from build123d import *

# Parameters (mm, degrees)
SKETCH1_W                     = 10.4775
SKETCH1_H                     = 12.7
SKETCH1_R                     = 2
SKETCH1_W_2                   = 13.97
BOSS_EXTRUDE1_DEPTH           = 7.9375
SKETCH2_W                     = 13.97
SKETCH2_H                     = 12.7
BOSS_EXTRUDE2_DEPTH           = 11.1125
CUT_EXTRUDE1_DEPTH            = 11.43
SKETCH4_R                     = 1.143
CUT_EXTRUDE2_DEPTH            = 32.637086722
CBORE_FOR_M4_SHCS1_AT_2_COUNT = 2
CBORE_FOR_M4_SHCS1_AT_2_PITCH = 24.4475
SKETCH8_R                     = 3
SKETCH8_R_2                   = 1.143
CUT_EXTRUDE3_DEPTH            = 32.637086722


with BuildPart() as part:
    # Sketch1 → Boss-Extrude1 (new body)
    # profile 1 of 5: a face of its own
    with BuildSketch(Plane.XY):
        with Locations((12.22375, 0)):
            Rectangle(SKETCH1_W, SKETCH1_H)
        with Locations((12.22375, 0)):
            Circle(SKETCH1_R, mode=Mode.SUBTRACT)
    # profile 2 of 5: a face of its own
    with BuildSketch(Plane.XY):
        Rectangle(SKETCH1_W_2, SKETCH1_H)
    # profile 3 of 5: a face of its own
    with BuildSketch(Plane.XY):
        with Locations((-12.22375, 0)):
            Rectangle(SKETCH1_W, SKETCH1_H)
        with Locations((-12.22375, 0)):
            Circle(SKETCH1_R, mode=Mode.SUBTRACT)
    # profile 4 of 5: a face of its own
    with BuildSketch(Plane.XY):
        with Locations((12.22375, 0)):
            Circle(SKETCH1_R)
    # profile 5 of 5: a face of its own
    with BuildSketch(Plane.XY):
        with Locations((-12.22375, 0)):
            Circle(SKETCH1_R)
    extrude(amount=BOSS_EXTRUDE1_DEPTH)

    # Sketch2 → Boss-Extrude2 (add)
    with BuildSketch(Plane.XY.offset(7.9375)):
        Rectangle(SKETCH2_W, SKETCH2_H)
    extrude(amount=BOSS_EXTRUDE2_DEPTH)

    # Sketch3 → Cut-Extrude1 (cut)
    with BuildSketch(Plane(origin=(6.985, 0, 0), x_dir=(0, 0, -1), z_dir=(1, 0, 0))):
        with BuildLine():
            ThreePointArc((-13.49375, 3), (-16.49375, 0), (-13.49375, -3))
            Line((-13.49375, -3), (-13.49375, -1.143))
            ThreePointArc((-13.49375, -1.143), (-14.63675, 0), (-13.49375, 1.143))
            Line((-13.49375, 1.143), (-13.49375, 3))
        make_face()
        with BuildLine():
            Line((-13.49375, -1.143), (-13.49375, -3))
            ThreePointArc((-13.49375, -3), (-11.372429656, -2.121320344), (-10.49375, 0))
            ThreePointArc((-10.49375, 0), (-11.372429656, 2.121320344), (-13.49375, 3))
            Line((-13.49375, 3), (-13.49375, 1.143))
            ThreePointArc((-13.49375, 1.143), (-12.685526949, 0.808223051), (-12.35075, 0))
            ThreePointArc((-12.35075, 0), (-12.685526949, -0.808223051), (-13.49375, -1.143))
        make_face()
        with BuildLine():
            ThreePointArc((-13.49375, 1.143), (-14.63675, 0), (-13.49375, -1.143))
            Line((-13.49375, -1.143), (-13.49375, 1.143))
        make_face()
        with BuildLine():
            Line((-13.49375, 1.143), (-13.49375, -1.143))
            ThreePointArc((-13.49375, -1.143), (-12.685526949, -0.808223051), (-12.35075, 0))
            ThreePointArc((-12.35075, 0), (-12.685526949, 0.808223051), (-13.49375, 1.143))
        make_face()
    extrude(amount=-CUT_EXTRUDE1_DEPTH, mode=Mode.SUBTRACT)

    # Sketch4 → Cut-Extrude2 (cut, through all)
    with BuildSketch(Plane(origin=(6.985, 0, 0), x_dir=(0, 0, -1), z_dir=(1, 0, 0))):
        with Locations((-13.49375, 0)):
            Circle(SKETCH4_R)
    extrude(amount=-CUT_EXTRUDE2_DEPTH, mode=Mode.SUBTRACT)

    # Sketch6 → CBORE for M4 SHCS1 (revolve, cut)
    with BuildSketch(Plane(origin=(12.22375, 0, 7.9375), x_dir=(0, -1, 0), z_dir=(1, 0, 0))):
        Polygon((0, 0), (0, 7.9375), (2.25, 7.9375), (2.25, 4), (4, 4), (4, 0.025), (4.025, 0), align=None)
    cbore_for_m4_shcs1 = revolve(axis=Axis((12.22375, 0, 14.2875), (0, 0, -1)), mode=Mode.SUBTRACT)

    # CBORE for M4 SHCS1 at 2: CBORE for M4 SHCS1 ×2
    with Locations(*[(-i * CBORE_FOR_M4_SHCS1_AT_2_PITCH, 0, 0) for i in range(1, CBORE_FOR_M4_SHCS1_AT_2_COUNT)]):
        add(cbore_for_m4_shcs1, mode=Mode.SUBTRACT)

    # Sketch8 → Cut-Extrude3 (cut, through all)
    # profile 1 of 2: a face of its own
    with BuildSketch(Plane(origin=(6.985, 0, 0), x_dir=(0, 0, -1), z_dir=(1, 0, 0))):
        with Locations((-13.49375, 0)):
            Circle(SKETCH8_R)
        with Locations((-13.49375, 0)):
            Circle(SKETCH8_R_2, mode=Mode.SUBTRACT)
    # profile 2 of 2: a face of its own
    with BuildSketch(Plane(origin=(6.985, 0, 0), x_dir=(0, 0, -1), z_dir=(1, 0, 0))):
        with Locations((-13.49375, 0)):
            Circle(SKETCH8_R_2)
    extrude(amount=-CUT_EXTRUDE3_DEPTH, mode=Mode.SUBTRACT)


solid = part.part
Verification items for the finished model (mm, model axes). A direction names the side the tool comes from. Give positions to 0.01 mm unless a question says otherwise; leave off trailing zeros. Order: outer loops, then holes, each group sorted by start corner. A loop starts at its lowest first (then second) coordinate and runs counter-clockwise, first axis right, second up. Notation, with made-up numbers: M 70.5,42.25 L 89.5,42.25 A27 cw 89.5,66.25 Z; hole C 60,-24 d6. An arc over 180 degrees is marked long. Answer as a JSON object with one key per item and string values. Group by question number.
1) Mould release check, pull along X, two halves, no side actions. Record for faces 6 (the face through (-17.462, 0, 4)), 7 (the face through (-10.5, 1.7, 3.938)), 8 (the face through (0, 0, 19.05)): released by +X, released by -X, zero draft, split by the parting line, or undercut.
2) Cross-section at C-C (z = 15.5). Enter the section's corners in (x, y) (3 decimals).
3) Scan lines: line 1 along X through (y, z) = (0, 5.25); line 2 along Z through (x, y) = (11, 3.5); line 3 along Y through (x, z) = (5, 14.5). Record each from-to range of solid material in increasing order. Write a range as [from, to].
4) Cross-section at B-B (x = -0.5). Enter the section's corners in (y, z), then the cut area to 3 significant figures.
5) Access from +Z, -Z, +X, -X, +Y, -Y to the whole of each face (thin tool, end or side, straight path). Record for faces 1 (the face through (12.2, 4.3, 7.938)), 2 (the face through (16.13, 0.87, 5.95)), 3 (the face through (17.462, 0, 4)), 4 (the face through (0, 0, 0)), 5 (the face through (-6.985, -3, 12)).
6) Cross-section at D-D (z = 7.5). Enter the section's corners in (x, y), then the cut area to 3 significant figures.
7) Depth check by flat-ended pin: pin 1 Ø5 at (x, y) = (-13.5, 3) entering from +Z; pin 2 Ø2.5 at (x, y) = (14, 2) entering from +Z. Enter the tip coordinate at first touch or a pass-through.
Result sheet:
{
 "1": {"face 6": "released by -X", "face 7": "undercut", "face 8": "zero draft"},
 "2": {"outline": "M -6.985,-6.35 L 6.985,-6.35 L 6.985,-2.23 L -6.985,-2.23 Z; M -6.985,2.23 L 6.985,2.23 L 6.985,6.35 L -6.985,6.35 Z"},
 "3": {"line 1": "x = [-17.46, -16.22], [-8.22, 8.22], [16.22, 17.46]", "line 2": "z = [0, 3.94]", "line 3": "y = [-6.35, -2.83], [2.83, 6.35]"},
 "4": {"outline": "M -6.35,0 L 6.35,0 L 6.35,19.05 L -6.35,19.05 Z; hole C 0,13.49 d6", "area": "214 mm2"},
 "5": {"face 1": "+Z, +X, +Y, -Y", "face 2": "+Z", "face 3": "+Z, -Z, +X, +Y, -Y", "face 4": "-Z, +X, -X, +Y, -Y", "face 5": "+Z, -X, +Y, -Y"},
 "6": {"outline": "M -17.46,-6.35 L 17.46,-6.35 L 17.46,6.35 L -17.46,6.35 Z; hole C -12.22,0 d8; hole C 12.22,0 d8", "area": "343 mm2"},
 "7": {"pin 1": "stops at z = 7.94", "pin 2": "stops at z = 3.94"}
}
